```python
from build123d import *

# Parameters (mm, degrees)
SKETCH1_W           = 30
SKETCH1_H           = 30
BOSS_EXTRUDE1_DEPTH = 30
SKETCH2_R           = 9
BOSS_EXTRUDE2_DEPTH = 235
SKETCH3_W           = 30
SKETCH3_H           = 30
BOSS_EXTRUDE3_DEPTH = 50
SKETCH4_W           = 30
SKETCH4_H           = 15
CUT_EXTRUDE1_DEPTH  = 40
SKETCH5_R           = 7.5
BOSS_EXTRUDE4_DEPTH = 15
FILLET1_R           = 7.5


with BuildPart() as part:
    # Sketch1 → Boss-Extrude1 (new body)
    with BuildSketch(Plane(origin=(0, 0, 0), x_dir=(1, 0, 0), z_dir=(0, 1, 0))):
        Rectangle(SKETCH1_W, SKETCH1_H)
    extrude(amount=BOSS_EXTRUDE1_DEPTH)

    # Sketch2 → Boss-Extrude2 (add)
    with BuildSketch(Plane(origin=(0, 30, 0), x_dir=(1, 0, 0), z_dir=(0, 1, 0))):
        Circle(SKETCH2_R)
    extrude(amount=BOSS_EXTRUDE2_DEPTH)

    # Sketch3 → Boss-Extrude3 (add)
    with BuildSketch(Plane(origin=(0, 265, 0), x_dir=(1, 0, 0), z_dir=(0, 1, 0))):
        Rectangle(SKETCH3_W, SKETCH3_H)
    extrude(amount=BOSS_EXTRUDE3_DEPTH)

    # Sketch4 → Cut-Extrude1 (cut)
    with BuildSketch(Plane(origin=(0, 315, 0), x_dir=(1, 0, 0), z_dir=(0, 1, 0))):
        Rectangle(SKETCH4_W, SKETCH4_H)
    extrude(amount=-CUT_EXTRUDE1_DEPTH, mode=Mode.SUBTRACT)

    # Sketch5 → Boss-Extrude4 (add)
    with BuildSketch(Plane(origin=(0, 0, 7.5), x_dir=(-1, 0, 0), z_dir=(0, 0, -1))):
        with Locations((0, 302.5)):
            Circle(SKETCH5_R)
    extrude(amount=BOSS_EXTRUDE4_DEPTH)

    # Fillet1
    fillet1_edges = [part.edges().sort_by_distance(p)[0] for p in [
        (15, 315, 11.25),
        (-15, 315, -11.25),
        (15, 315, -11.25),
        (-15, 315, 11.25),
    ]]
    fillet(fillet1_edges, radius=FILLET1_R)


solid = part.part
```
CAD build for the part. Positions are in the model's coordinates, mm. A direction names the side the tool comes from. Round coordinates to 2 decimals unless told otherwise and drop trailing zeros. Order: outer loops, then holes, each group sorted by start corner. A loop starts at its lowest first (then second) coordinate and runs counter-clockwise, first axis right, second up.
Q1. Drop flat-ended pins along their axis: pin 1 (3 mm diameter, centred on y = 189.5, z = -4, fed in from -X); pin 2 (4.5 mm diameter, centred on x = 2.5, z = -3, fed in from +Y); pin 3 (6 mm diameter, centred on x = 11.5, z = 10.5, fed in from +Y). Give the stop position or say it passes through.
Q2. Two-plate mould, pull along Z, no slides. Class faces 1 (the flat face through (-15, 281, 10)), 2 (the flat face through (0, 275, 0)), 3 (the flat face through (0, 15, -15)), 4 (the flat face through (0, 291, 7.5)): pulls with the +Z half, pulls with the -Z half, needs draft (parallel to the pull), parting line crosses it, or undercut.
Q3. Slice it at C-C (y = 139.5). Write the cut outline in (x, z), and give its area (3 significant figures).
Q4. Slice it at A-A (y = 281). Write the cut outline in (x, z).
Q5. Which spindle directions (+Z, -Z, +X, -X, +Y, -Y) get a long thin tool onto all of the face, cutting with end or side? Do faces 5 (the flat face through (-15, 15, 0)), 6 (the flat face through (-7, 265, -7)). Say none if no direction does.
Q6. Wall check: L1, parallel to Y at x = -10.5, z = -1; L2, parallel to Y at x = 6.5, z = -13; L3, parallel to X at y = 46, z = -1. Give the ranges that are in metal, low to high.
Q7. Slice it at B-B (x = 0). Write the cut outline in (y, z), and give its area (4 significant figures).
Results below:
1. pin 1: stops at x = -8.65
1. pin 2: stops at y = 310
1. pin 3: stops at y = 314.93
2. face 1: needs draft
2. face 2: undercut
2. face 3: pulls with the -Z half
2. face 4: undercut
3. outline: circle Ø18 at (0, 0)
3. area: 254 mm2
4. outline: (-15, -15) - (15, -15) - (15, -7.5) - (-15, -7.5) - close; (-15, 7.5) - (15, 7.5) - (15, 15) - (-15, 15) - close
5. face 5: +Z, -Z, -X, +Y, -Y
5. face 6: none
6. L1: y = 0 to 30, 265 to 275
6. L2: y = 0 to 30, 265 to 315
6. L3: x = -8.94 to 8.94
7. outline: (0, -15) - (30, -15) - (30, -9) - (265, -9) - (265, -15) - (315, -15) - (315, -7.5) - (310, -7.5) - (310, 7.5) - (315, 7.5) - (315, 15) - (265, 15) - (265, 9) - (30, 9) - (30, 15) - (0, 15) - close; hole (275, -7.5) - (295, -7.5) - (295, 7.5) - (275, 7.5) - close
7. area: 6,255 mm2
